from build123d import *

# Parameters (mm, degrees)
SKETCH_W        = 30
SKETCH_H        = 20
PAD_DEPTH       = 5
SKETCH001_R     = 1.2
POCKET_DEPTH    = 5
SKETCH002_R     = 2.65
POCKET001_DEPTH = 5


with BuildPart() as part:
    # Sketch → Pad (new body)
    with BuildSketch(Plane.XY):
        Rectangle(SKETCH_W, SKETCH_H)
    extrude(amount=PAD_DEPTH)

    # Sketch001 (on Face6 of Pad) → Pocket (cut)
    with BuildSketch(Plane.XY.offset(5)):
        with Locations((8, 5)):
            Circle(SKETCH001_R)
        with Locations((8, -5)):
            Circle(SKETCH001_R)
    extrude(amount=-POCKET_DEPTH, mode=Mode.SUBTRACT)

    # Sketch002 (on Face5 of Pocket) → Pocket001 (cut)
    with BuildSketch(Plane.XY.offset(5)):
        with Locations((-7.5, 0)):
            Circle(SKETCH002_R)
    extrude(amount=-POCKET001_DEPTH, mode=Mode.SUBTRACT)


solid = part.part
For this review, take the finished solid that the model builds, in its own axes (mm). Coordinates: 2 decimals unless noted, no trailing zeros. Loops run counter-clockwise (first coordinate to the right, second up) from the corner with the lowest first, then second, coordinate; pieces in that order, holes last. Notation, with made-up numbers: (61.5, 58) - (71.5, 58) arc R22 ccw to (71.5, 93) - close; hole circle Ø10 at (52, 74.25). An arc over 180 degrees is marked (long way). Use a Markdown table: item, result. Add a question column.
Item 1: For line 1 (Y direction, x = 8.75, z = 3.6); line 2 (X direction, y = 1.5, z = 3.15); line 3 (Y direction, x = -7.5, z = 2.3), list the stretches that pass through material, from the lowest coordinate up.
Item 2: We need section D-D (y = -1.5). Give the boundary of the cut face in (x, z), and give its area (3 significant figures).
Item 3: We need section A-A (x = 8). Give the boundary of the cut face in (y, z), and give its area (3 significant figures).
Item 4: We need section B-B (y = -5). Give the boundary of the cut face in (x, z).
Item 5: Mouldability with a two-part tool opening along X and no side actions: class faces 1 (the face through (0, 0, 0)), 2 (the face through (-15, 0, 2)), 3 (the face through (-10.147, 0.117, 2.535)), 4 (the face through (6.8, -4.95, 2.54)) as pulls with the +X half, pulls with the -X half, needs draft (parallel to the pull), parting line crosses it, or undercut.
Item 6: We need section C-C (z = 0.5). Give the boundary of the cut face in (x, y), and give its area (3 significant figures).
Results list:
| question | item | result |
|---|---|---|
| 1 | line 1 | y = -10 to -5.94, -4.06 to 4.06, 5.94 to 10 |
| 1 | line 2 | x = -15 to -9.68, -5.32 to 15 |
| 1 | line 3 | y = -10 to -2.65, 2.65 to 10 |
| 2 | outline | (-15, 0) - (-9.68, 0) - (-9.68, 5) - (-15, 5) - close; (-5.32, 0) - (15, 0) - (15, 5) - (-5.32, 5) - close |
| 2 | area | 128 mm^2 |
| 3 | outline | (-10, 0) - (-6.2, 0) - (-6.2, 5) - (-10, 5) - close; (-3.8, 0) - (3.8, 0) - (3.8, 5) - (-3.8, 5) - close; (6.2, 0) - (10, 0) - (10, 5) - (6.2, 5) - close |
| 3 | area | 76.0 mm^2 |
| 4 | outline | (-15, 0) - (6.8, 0) - (6.8, 5) - (-15, 5) - close; (9.2, 0) - (15, 0) - (15, 5) - (9.2, 5) - close |
| 5 | face 1 | needs draft |
| 5 | face 2 | pulls with the -X half |
| 5 | face 3 | undercut |
| 5 | face 4 | undercut |
| 6 | outline | (-15, -10) - (15, -10) - (15, 10) - (-15, 10) - close; hole circle Ø5.3 at (-7.5, 0); hole circle Ø2.4 at (8, -5); hole circle Ø2.4 at (8, 5) |
| 6 | area | 569 mm^2 |
